Autodesk Inventor part; units mm, degrees
ref_plane "Work Plane1" through (0, 0, 0) normal (0, 0, 1) x (1, 0, 0)
ref_plane "YZ Plane" through (0, 0, 0) normal (1, 0, 0) x (0, 1, 0)
ref_plane "XZ Plane" through (0, 0, 0) normal (0, 1, 0) x (-1, 0, 0)
ref_plane "Work Plane1" through (0, 0, 0) normal (0, 0, 1) x (1, 0, 0)
sketch "mount_sketch" plane through (0, 0, 0) normal (0, 0, 1) x (1, 0, 0)
  circle A0 centre (42, 55.2584) radius 1.55
  circle A1 centre (28, 55.2584) radius 1.55
  line L0 (45, 60.2584) -> (25, 60.2584)
  line L1 (25, 60.2584) -> (15.4, 52.7584)
  line L2 (15.4, 52.7584) -> (15.4, 29.5584)
  line L3 (15.4, 29.5584) -> (19.4, 29.5584)
  line L4 (19.4, 29.5584) -> (19.4, 48.7584)
  line L5 (19.4, 48.7584) -> (23, 48.7584)
  circle A2 centre (42, -54.7416) radius 1.55 construction
  circle A3 centre (28, -54.7416) radius 1.55 construction
  line L6 (47, -54.627) -> (47, 66.2497) construction
  circle A4 centre (12, 51.2584) radius 1.55 construction
  circle A5 centre (12, -37.8416) radius 1.55 construction
  circle A6 centre (12, -54.7416) radius 1.55 construction
  circle A7 centre (29, -68.7416) radius 1.55 construction
  circle A8 centre (14, -68.7416) radius 1.55 construction
  line L7 (45, 50.2584) -> (25, 50.2584)
  line L8 (25, 50.2584) -> (23, 48.7584)
  line L9 (45, 60.2584) -> (46.5, 60.2584)
  line L10 (46.5, 60.2584) -> (46.5, 50.2584)
  line L11 (46.5, 50.2584) -> (45, 50.2584)
  line L12 (23, 48.7584) -> (23, 58.6959)
  line L13 (35, 55.2584) -> (35, 60.2584)
  line L14 (35, 55.2584) -> (35, 50.2584)
  line L15 (46.5, 60.2584) -> (46.6, 60.2584)
  line L16 (46.6, 60.2584) -> (46.6, 50.2584)
  line L17 (46.6, 50.2584) -> (46.5, 50.2584)
  line L18 (46.6, 60.2584) -> (50.6, 60.2584)
  line L19 (50.6, 60.2584) -> (50.6, 50.2584)
  line L20 (50.6, 50.2584) -> (46.6, 50.2584)
  line L21 (46.6, 50.2584) -> (46.6, 60.2584)
  line L22 (48.1, 58.7584) -> (49.1, 58.7584)
  line L23 (49.1, 58.7584) -> (49.1, 51.7584)
  line L24 (49.1, 51.7584) -> (48.1, 51.7584)
  line L25 (48.1, 51.7584) -> (48.1, 58.7584)
  point P0 (0, 0)
  dimension "d1" = 110
  dimension "d2" = 6.5
  dimension "d3" = 27.6
  dimension "d4" = 4
  dimension "d5" = 14
  dimension "d6" = 5
  dimension "d7" = 19.2
  dimension "d9" = 3.4
  dimension "d13" = 3
  dimension "d30" = 2
  dimension "d32" = 5
  dimension "d62" = 4.5
  dimension "d77" = 4.6
  dimension "d128" = 4
  dimension "d129" = 1.5
  dimension "d130" = 1.5
  dimension "d132" = 7
  dimension "d133" = 1.5
extrude "mount" add sketch "mount_sketch" along normal blind 6
fillet "common" radius 2 2 edges at (25, 60.2584, 3) (25, 50.2584, 3)
sketch "nuts_sketch" plane through (0, 0, 6) normal (0, 0, 1) x (1, 0, 0)
  circle A0 centre (42, 55.2584) radius 1.55
  circle A1 centre (28, 55.2584) radius 1.55
  line L0 (38.4782, 55.2584) -> (40.2391, 58.3084)
  line L1 (40.2391, 58.3084) -> (43.7609, 58.3084)
  line L2 (43.7609, 58.3084) -> (45.5218, 55.2584)
  line L3 (45.5218, 55.2584) -> (43.7609, 52.2084)
  line L4 (43.7609, 52.2084) -> (40.2391, 52.2084)
  line L5 (40.2391, 52.2084) -> (38.4782, 55.2584)
  line L6 (31.5218, 55.2584) -> (29.7609, 52.2084)
  line L7 (29.7609, 52.2084) -> (26.2391, 52.2084)
  line L8 (26.2391, 52.2084) -> (24.4782, 55.2584)
  line L9 (24.4782, 55.2584) -> (26.2391, 58.3084)
  line L10 (26.2391, 58.3084) -> (29.7609, 58.3084)
  line L11 (29.7609, 58.3084) -> (31.5218, 55.2584)
  point P0 (0, 0)
  dimension "d26" = 6.1
  dimension "d27" = 6.1
extrude "nuts" cut sketch "nuts_sketch" against normal blind 3
sketch "Sketch20" plane through (19.4, 29.5584, 0) normal (1, 0, 0) x (0, 0, -1)
  line L0 (-6, 0) -> (-6, 19.2)
  line L1 (-6, 0) -> (-6, 19.2)
  line L2 (0, 19.2) -> (-6, 19.2)
  line L3 (-6, 19.2) -> (0, 19.2)
  line L4 (0, 0) -> (-6, 0)
  line L5 (0, 19.2) -> (0, 0)
  line L6 (0, 0) -> (-6, 0)
  point P0 (0, -29.5584)
extrude "Extrusion15" add sketch "Sketch20" along normal blind 3.6
sketch "Sketch21" plane through (0, 0, 6) normal (0, 0, 1) x (1, 0, 0)
  line L0 (15.4, 29.5584) -> (23, 29.5584)
  line L1 (19.2, 29.5584) -> (19.2, 55.7272)
  line L2 (24.4573, 59.8345) -> (15.4, 52.7584)
  line L3 (15.4, 52.7584) -> (15.4, 29.5584)
  line L4 (19.2, 29.5584) -> (15.4, 29.5584)
  line L5 (15.4, 29.5584) -> (15.4, 52.7584)
  line L6 (15.4, 52.7584) -> (19.2, 55.7272)
  line L7 (23, 48.7584) -> (24.4667, 49.8584)
  line L8 (23, 48.7584) -> (19.2, 48.7584)
  line L9 (23, 48.7584) -> (23, 29.5584)
  line L10 (23, 48.7584) -> (23, 58.6959)
  line L11 (19.2, 48.7584) -> (23, 58.6959)
  point P0 (0, 0)
extrude "Extrusion16" cut sketch "Sketch21" against normal blind 6 contours L3 L2 L1 L0
sketch "Sketch22" plane through (0, 0, 6) normal (0, 0, 1) x (1, 0, 0)
  line L0 (23, 48.7584) -> (23, 29.5584)
  line L1 (23, 48.7584) -> (23, 58.6959)
  line L2 (24.4573, 59.8345) -> (19.2, 55.7272)
  line L3 (23, 48.7584) -> (19.2, 48.7584)
  line L4 (19.2, 29.5584) -> (19.2, 55.7272)
  point P0 (0, 0)
fillet "Fillet12" radius 10 1 edges at (19.2, 55.7272, 3)
fillet "Fillet13" radius 2 1 edges at (23, 48.7584, 3)
fillet "Fillet14" radius 2 2 edges at (23, 29.5584, 3) (19.2, 29.5584, 3)
sketch "Sketch28" plane through (0, 0, 6) normal (0, 0, 1) x (1, 0, 0)
  line L0 (24.4782, 55.2584) -> (26.2391, 58.3084)
  line L1 (26.2391, 58.3084) -> (29.7609, 58.3084)
  line L2 (29.7609, 58.3084) -> (31.5218, 55.2584)
  line L3 (31.5218, 55.2584) -> (29.7609, 52.2084)
  line L4 (29.7609, 52.2084) -> (26.2391, 52.2084)
  line L5 (26.2391, 52.2084) -> (24.4782, 55.2584)
  arc A0 (25.6886, 60.2584) -> (24.4573, 59.8345) centre (25.6886, 58.2584) ccw
  line L6 (24.4573, 59.8345) -> (23.0436, 58.73)
  arc A1 (23.0436, 58.73) -> (19.2, 50.8497) centre (29.2, 50.8497) ccw
  line L7 (19.2, 50.8497) -> (19.2, 31.5484)
  arc A2 (19.2, 31.5484) -> (21, 29.5584) centre (21.2, 31.5484) ccw
  arc A3 (21, 29.5584) -> (23, 31.5584) centre (21, 31.5584) ccw
  line L8 (23, 47.7584) -> (23, 31.5584)
  arc A4 (23.8, 49.3584) -> (23, 47.7584) centre (25, 47.7584) ccw
  line L9 (23.8, 49.3584) -> (24.4667, 49.8584)
  arc A5 (25.6667, 50.2584) -> (24.4667, 49.8584) centre (25.6667, 48.2584) ccw
  line L10 (45.5218, 55.2584) -> (43.7609, 52.2084)
  line L11 (43.7609, 52.2084) -> (40.2391, 52.2084)
  line L12 (40.2391, 52.2084) -> (38.4782, 55.2584)
  line L13 (38.4782, 55.2584) -> (40.2391, 58.3084)
  line L14 (40.2391, 58.3084) -> (43.7609, 58.3084)
  line L15 (43.7609, 58.3084) -> (45.5218, 55.2584)
  line L16 (29.7609, 52.2084) -> (26.2391, 52.2084)
  line L17 (26.2391, 52.2084) -> (19.2927, 52.2084)
  line L18 (24.4782, 55.2584) -> (22.3512, 55.2584)
  line L19 (22.3512, 55.2584) -> (22.3512, 52.823)
  line L20 (22.3512, 55.2584) -> (20.2243, 55.2584)
  line L21 (22.3512, 55.2584) -> (22.3512, 57.0751)
  line L22 (20.8512, 56.7584) -> (22.3512, 56.7584)
  line L23 (23.8512, 56.7584) -> (23.8512, 53.7584)
  line L24 (23.8512, 53.7584) -> (20.8512, 53.7584)
  line L25 (20.8512, 53.7584) -> (20.8512, 55.2584)
  line L26 (20.8512, 55.2584) -> (20.8512, 56.7584)
  line L27 (22.3512, 56.7584) -> (23.8512, 56.7584)
  line L28 (25.6667, 50.2584) -> (50.6, 50.2584)
  line L29 (50.6, 50.2584) -> (50.6, 60.2584)
  line L30 (50.6, 60.2584) -> (25.6886, 60.2584)
  point P0 (0, 0)
  dimension "d121" = 3
  dimension "d122" = 3
extrude "hook" add sketch "Sketch28" along normal blind 3 contours L23 L24 L19 L18 | L18 L21 L27 L23 | L19 L24 L25 L20 | L20 L26 A1 L22 L21 | L26 L22 A1
sketch "Sketch29" plane through (20.8512, 53.7584, 6) normal (0, -1, 0) x (1, 0, 0)
  line L0 (3, 0) -> (0, 0)
  line L1 (3, 0) -> (3, 3)
  line L2 (0, 3) -> (3, 3)
  line L3 (0, 0) -> (0, 3)
  line L4 (0, 0) -> (1.5, 0)
  line L5 (1.5, 0) -> (1.5, 1.7757)
  line L6 (1.5, 1.7757) -> (0, 1.7757)
  line L7 (0, 1.7757) -> (0, 0)
  line L8 (1.5, 1.7757) -> (3, 1.7757)
  line L9 (0, 0) -> (0, 3)
  line L10 (0, 1.7757) -> (0, 3)
  point P0 (-20.8512, -6)
extrude "hook_cutout" cut sketch "Sketch29" against normal through all contours L0 L3 L6 L5
sketch "Sketch33" plane through (0, 0, 6) normal (0, 0, 1) x (1, 0, 0)
  line L0 (49.1, 58.7584) -> (49.1, 51.7584)
  line L1 (49.1, 51.7584) -> (48.1, 51.7584)
  line L2 (48.1, 51.7584) -> (48.1, 58.7584)
  line L3 (48.1, 58.7584) -> (49.1, 58.7584)
  line L4 (25.6667, 50.2584) -> (50.6, 50.2584)
  line L5 (50.6, 60.2584) -> (25.6886, 60.2584)
  line L6 (50.6, 50.2584) -> (46.6, 50.2584)
  line L7 (46.6, 50.2584) -> (46.6, 60.2584)
  line L8 (46.6, 60.2584) -> (50.6, 60.2584)
  line L9 (50.6, 60.2584) -> (50.6, 50.2584)
  point P0 (0, 0)
  dimension "d141" = 4
extrude "Extrusion25" cut sketch "Sketch33" against normal blind 4.5
fillet "Fillet21" radius 0.75 9 edges at (49.1, 55.2584, 1.5) (50.6, 55.2584, 1.5) (49.1, 55.2584, 0) (50.6, 55.2584, 0) (46.6, 55.2584, 6) (20.8512, 55.2584, 9) (23.8512, 55.2584, 9) (20.8512, 56.7584, 8.3879) (20.8512, 53.7584, 8.3879)
equation "\"d27\" = d26"
equation "\"hook_width\" = 1.5"
equation "\"hook_height\" = 7"
properties part number "mount_battery" material "ABS Plastic"
Model file for the job. Use its own axes, mm. A direction names the side the tool comes from. Give positions to 0.01 mm unless a question says otherwise; leave off trailing zeros. Order: outer loops, then holes, each group sorted by start corner. A loop starts at its lowest first (then second) coordinate and runs counter-clockwise, first axis right, second up.
1) Saw through at B-B, the plane x = 39. Write the cut outline in (y, z), then the cut area to 3 significant figures.
2) Saw through at C-C, the plane x = 43. Write the cut outline in (y, z).
3) Wall check: probe 1 along Y at (x, z) = (28, 1.2); probe 2 along Y at (x, z) = (41, 5.5); probe 3 along X at (y, z) = (33, 4.5). Give the ranges that are in metal, low to high.
4) Mould opens along X. For faces 4 (the cylindrical face through (25.046, 60.152, 3.042)), 5 (the cylindrical face through (23.217, 48.664, 3.042)), 6 (the flat face through (42, 52.208, 5)), 7 (the flat face through (23, 56.758, 7)) say: +X half, -X half, draft (parallel to the pull), parting line (faces both ways), or undercut.
5) Pin check, flat tips, straight feed: pin 1 (6 mm diameter, centred on x = 32, y = 48, fed in from +Z); pin 2 (0.9 mm diameter, centred on x = 27.5, z = 5, fed in from -Y); pin 3 (2 mm diameter, centred on y = 55.5, z = 6.5, fed in from -X); pin 4 (1.6 mm diameter, centred on x = 22, y = 55, fed in from -Z). Stop position of each tip, or through.
6) 3-axis set-ups, long thin cutter, end or side, ignore diameter. For faces 1 (the flat face through (36, 50.258, 3)), 2 (the flat face through (42, 58.308, 5)), 3 (the flat face through (48.1, 55, 1)): which of +Z, -Z, +X, -X, +Y, -Y reach the whole face in a straight line?
7) Saw through at A-A, the plane x = 28. Write the cut outline in (y, z), then the cut area to 3 significant figures.
Computed:
1. outline: (50.26, 0) - (60.26, 0) - (60.26, 6) - (56.16, 6) - (56.16, 3) - (54.35, 3) - (54.35, 6) - (50.26, 6) - close
1. area: 54.6 mm2
2. outline: (50.26, 0) - (54.07, 0) - (54.07, 3) - (52.21, 3) - (52.21, 6) - (50.26, 6) - close; (56.44, 0) - (60.26, 0) - (60.26, 6) - (58.31, 6) - (58.31, 3) - (56.44, 3) - close
3. probe 1: y = 50.26 to 53.71, 56.81 to 60.26
3. probe 2: y = 50.26 to 52.21, 58.31 to 60.26
3. probe 3: x = 19.2 to 23
4. face 4: -X half
4. face 5: +X half
4. face 6: undercut
4. face 7: draft
5. pin 1: stops at z = 6
5. pin 2: stops at y = 50.26
5. pin 3: stops at x = 19.94
5. pin 4: stops at z = 0
6. face 1: +Z, -Z, +X, -Y
6. face 2: +Z
6. face 3: +Z, -Z
7. outline: (50.26, 0) - (53.71, 0) - (53.71, 3) - (52.21, 3) - (52.21, 6) - (50.26, 6) - close; (56.81, 0) - (60.26, 0) - (60.26, 6) - (58.31, 6) - (58.31, 3) - (56.81, 3) - close
7. area: 32.4 mm2
